```python
from build123d import *

# Parameters (mm, degrees)
BOSS_EXTRUDE1_DEPTH   = 1.25
F_4_CLEARANCE_HOLE1_D = 3.2639
SKETCH5_R             = 7.5
BOSS_EXTRUDE2_DEPTH   = 3.25
FILLET2_R             = 2


with BuildPart() as part:
    # Sketch1 → Boss-Extrude1 (new body)
    with BuildSketch(Plane(origin=(0, 0, 0), x_dir=(1, 0, 0), z_dir=(0, 1, 0))):
        Polygon((24, 0), (-12, 20.784609691), (-12, -20.784609691), align=None)
    extrude(amount=BOSS_EXTRUDE1_DEPTH)

    # #4 Clearance Hole1 (through all)
    with Locations(Plane(origin=(0, 1.25, 0), x_dir=(1, 0, 0), z_dir=(0, 1, 0))):
        with Locations((-8.5, 14.722431864), (-8.5, -14.722431864), (17, 0)):
            Hole(F_4_CLEARANCE_HOLE1_D / 2)

    # Sketch4 → Revolve1 (revolve)
    with BuildSketch(Plane(origin=(0, 0, 0), x_dir=(0, 0, -1), z_dir=(1, 0, 0)), mode=Mode.PRIVATE) as revolve1_sk:
        Polygon((0, 1.25), (6, 1.25), (6, 3.75), (14, 3.75), (14, 21.75), (4, 21.75), (4, 30.75), (5.5, 30.75), (5.5, 31.5), (2.3, 31.5), (2.3, 44.5), (0, 44.5), align=None)
    revolve(revolve1_sk.sketch.rotate(Axis((0, 44.5, 0), (0, -1, 0)), 180), axis=Axis((0, 44.5, 0), (0, -1, 0)))

    # Sketch5 → Boss-Extrude2 (add)
    with BuildSketch(Plane.XZ):
        with Locations(Location((0, 0, 0), (0, 0, 90))):
            Circle(SKETCH5_R)
    extrude(amount=BOSS_EXTRUDE2_DEPTH)

    # Fillet2
    fillet2_edges = [part.edges().sort_by_distance(p)[0] for p in [
        (-12, 0.625, 20.784609691),
        (-12, 0.625, -20.784609691),
        (24, 0.625, 0),
    ]]
    fillet(fillet2_edges, radius=FILLET2_R)


solid = part.part
```
The listing builds one solid part. Answer for the finished solid, in the listing's coordinates (mm). A direction names the side the tool comes from. Give positions to 0.01 mm unless a question says otherwise; leave off trailing zeros. Order: outer loops, then holes, each group sorted by start corner. A loop starts at its lowest first (then second) coordinate and runs counter-clockwise, first axis right, second up. Notation, with made-up numbers: M -22,-8.75 L 9,-8.75 A34 ccw 9,21.25 Z; hole C 30.25,50 d2. An arc over 180 degrees is marked long. Put each result on its own line as item: value. Start each with the question number.
Item 1: Flat-ended cylindrical pins translate along their axes: P1, Ø4, axis at x = -2.5, y = 32, coming from the +Z side; P2, Ø4, axis at x = 17, z = 0, coming from the +Y side; P3, Ø4, axis at x = 13, y = 21.5, coming from the +Z side. Find the tip coordinate at first contact, or state that the pin passes through.
Item 2: Find the intervals of material crossed by line 1 along Z through (x, y) = (-8.5, 0.75); line 2 along Y through (x, z) = (3.5, 8.5); line 3 along Y through (x, z) = (9, 10), in increasing order.
Item 3: Which of the six approach directions +Z, -Z, +X, -X, +Y, -Y give full straight-line access (tool end or side, diameter ignored) to faces 1 (the face through (6.21, 0.62, -10.27)), 2 (the face through (6, 3.75, -3)), 3 (the face through (-12, 1, 0))?
Item 4: The part is cut by section D-D, the plane x = 0. Determine the outline of the cut face in (y, z), and give its area (3 significant figures).
Item 5: The part is cut by section B-B, the plane x = 17. Determine the outline of the cut face in (y, z), and give its area (3 significant figures).
Item 6: For a pull along Y with two mould halves and no side action, classify faces 4 (the face through (0, 44.5, 0)), 5 (the face through (-0.33, -1.602, -7.493)), 6 (the face through (-7, 0, 4)), 7 (the face through (-1.802, 2.518, 5.723)) as +Y half, -Y half, draft (parallel to the pull), parting line (faces both ways), or undercut.
Item 7: The part is cut by section C-C, the plane y = 39. Determine the outline of the cut face in (x, z).
Answer key:
1. P1: stops at z = 5.47
1. P2: stops at y = 1.25
1. P3: stops at z = 8.66
2. line 1: z = -18.76 to -16.35, -13.09 to 13.09, 16.35 to 18.76
2. line 2: y = 0 to 1.25, 3.75 to 21.75
2. line 3: y = 3.75 to 21.75
3. face 1: -Z, +X, -Y
3. face 2: none
3. face 3: +Z, -Z, -X, -Y
4. outline: M -3.25,-7.5 L 0,-7.5 L 0,-13.86 L 1.25,-13.86 L 1.25,-6 L 3.75,-6 L 3.75,-14 L 21.75,-14 L 21.75,-4 L 30.75,-4 L 30.75,-5.5 L 31.5,-5.5 L 31.5,-2.3 L 44.5,-2.3 L 44.5,2.3 L 31.5,2.3 L 31.5,5.5 L 30.75,5.5 L 30.75,4 L 21.75,4 L 21.75,14 L 3.75,14 L 3.75,6 L 1.25,6 L 1.25,13.86 L 0,13.86 L 0,7.5 L -3.25,7.5 Z
4. area: 757 mm²
5. outline: M 0,-4.04 L 1.25,-4.04 L 1.25,-1.63 L 0,-1.63 Z; M 0,1.63 L 1.25,1.63 L 1.25,4.04 L 0,4.04 Z
5. area: 6.02 mm²
6. face 4: +Y half
6. face 5: draft
6. face 6: -Y half
6. face 7: undercut
7. outline: C 0,0 d4.6
